The listing builds one solid part. Answer for the finished solid, in the listing's coordinates (mm). A direction names the side the tool comes from. Give positions to 0.01 mm unless a question says otherwise; leave off trailing zeros. Order: outer loops, then holes, each group sorted by start corner. A loop starts at its lowest first (then second) coordinate and runs counter-clockwise, first axis right, second up. Notation, with made-up numbers: (56.25, 1.25) - (91.25, 1.25) arc R21 ccw to (91.25, 22.25) - close; hole circle Ø7 at (52, -4). An arc over 180 degrees is marked (long way). Answer in a Markdown table with one row per item. Add a question column.
```python
from build123d import *

# Parameters (mm, degrees)
AUFSATZ_LINEAR_AUSTRAGEN1_DEPTH = 50
SKIZZE3_R                       = 1.25
SKIZZE3_R_2                     = 1.5
SCHNITT_LINEAR_AUSTRAGEN1_DEPTH = 3
SKIZZE4_W                       = 5
SKIZZE4_H                       = 44
SCHNITT_LINEAR_AUSTRAGEN2_DEPTH = 27
SKIZZE5_R                       = 2.5
SCHNITT_LINEAR_AUSTRAGEN3_DEPTH = 28
SKIZZE6_R                       = 1.25
SCHNITT_LINEAR_AUSTRAGEN4_DEPTH = 3
SKIZZE7_W                       = 5
SKIZZE7_H                       = 15
SCHNITT_LINEAR_AUSTRAGEN5_DEPTH = 3


with BuildPart() as part:
    # Skizze2 → Aufsatz-Linear austragen1 (new body)
    with BuildSketch(Plane.XY):
        Polygon((-4.170146195, 14.050114253), (-21.49065427, -15.949885747), (13.50934573, -15.949885747), (13.50934573, 14.050114253), align=None)
        Polygon((5.50934573, -12.949885747), (-16.294501848, -12.949885747), (-2.438095387, 11.050114253), (5.50934573, 11.050114253), align=None, mode=Mode.SUBTRACT)
    extrude(amount=AUFSATZ_LINEAR_AUSTRAGEN1_DEPTH)

    # Skizze3 → Schnitt-Linear austragen1 (cut)
    with BuildSketch(Plane.XZ.offset(15.949885747)):
        with Locations((11.00934573, 40)):
            Circle(SKIZZE3_R)
        with Locations((11.00934573, 10)):
            Circle(SKIZZE3_R)
        with Locations((1.00934573, 41.25)):
            Circle(SKIZZE3_R_2)
        with Locations((1.00934573, 8.75)):
            Circle(SKIZZE3_R_2)
    extrude(amount=-SCHNITT_LINEAR_AUSTRAGEN1_DEPTH, mode=Mode.SUBTRACT)

    # Skizze4 → Schnitt-Linear austragen2 (cut)
    with BuildSketch(Plane(origin=(0, 14.050114253, 0), x_dir=(1, 0, 0), z_dir=(0, 1, 0))):
        with Locations((11.00934573, -25)):
            Rectangle(SKIZZE4_W, SKIZZE4_H)
    extrude(amount=-SCHNITT_LINEAR_AUSTRAGEN2_DEPTH, mode=Mode.SUBTRACT)

    # Skizze5 → Schnitt-Linear austragen3 (cut)
    with BuildSketch(Plane(origin=(0, 14.050114253, 0), x_dir=(1, 0, 0), z_dir=(0, 1, 0))):
        with Locations((1.00934573, -41.25)):
            Circle(SKIZZE5_R)
        with Locations((1.00934573, -8.75)):
            Circle(SKIZZE5_R)
    extrude(amount=-SCHNITT_LINEAR_AUSTRAGEN3_DEPTH, mode=Mode.SUBTRACT)

    # Skizze6 → Schnitt-Linear austragen4 (cut)
    with BuildSketch(Plane(origin=(-9.21148758, 5.318254834, 0), x_dir=(0, 0, 1), z_dir=(-0.866025404, 0.5, 0))):
        with Locations((35, -1.917317229)):
            Circle(SKIZZE6_R)
        with Locations((15, -1.917317229)):
            Circle(SKIZZE6_R)
    extrude(amount=-SCHNITT_LINEAR_AUSTRAGEN4_DEPTH, mode=Mode.SUBTRACT)

    # Skizze7 → Schnitt-Linear austragen5 (cut)
    with BuildSketch(Plane(origin=(-9.21148758, 5.318254834, 0), x_dir=(0, 0, 1), z_dir=(-0.866025404, 0.5, 0))):
        with Locations((47.5, -7.05833338)):
            Rectangle(SKIZZE7_W, SKIZZE7_H)
        with Locations((2.5, -7.05833338)):
            Rectangle(SKIZZE7_W, SKIZZE7_H)
    extrude(amount=-SCHNITT_LINEAR_AUSTRAGEN5_DEPTH, mode=Mode.SUBTRACT)


solid = part.part
```
(1) Each of these flat-tipped pins is pushed along its axis until it touches: P1, Ø6, axis at x = -12, z = 29, coming from the +Y side; P2, Ø4, axis at y = 8, z = 40, coming from the -X side; P3, Ø2.5, axis at x = 1.5, z = 41.5, coming from the +Y side. Where does it stop, or does it pass through?
(2) Straight lines are drawn through the part: line 1 (Y direction, x = 1, z = 5.5); line 2 (X direction, y = -14, z = 41); line 3 (Z direction, x = 12, y = 9). For each, find the intervals that lie inside material, in ascending order.
(3) Find section A-A, the plane z = 29. Write down the section's boundary in (x, y), plus the area to 3 significant figures.
(4) Find section D-D, the plane x = 0.5. Give the number of separate pieces and of enclosed holes in the cut face, plus the area to 3 significant figures.
(5) Find section B-B, the plane y = -3. Write down the section's boundary in (x, z), plus the area to 3 significant figures.
(6) For faces 4 (the face through (-7.71, 4.96, 2.47)), 5 (the face through (0.47, -13.44, 43.69)), 6 (the face through (-15.21, -8.03, 2.47)), 7 (the face through (-7.71, 4.96, 47.46)), 8 (the face through (-9.463, -1.118, 24.65)), determine the directions among +Z, -Z, +X, -X, +Y, -Y from which every point of the face is accessible in a straight line to the end or side of a thin tool.
(7) Find section C-C, the plane x = 10.5. Write down the section's boundary in (y, z).
(8) The mould has two halves that part along X. Classify faces 1 (the face through (11, 1, 47)), 2 (the face through (13.509, -13.2, 24.9)), 3 (the face through (0.684, -14.964, 7.286)): +X half, -X half, draft (parallel to the pull), parting line (faces both ways), or undercut.
Answer key:
| question | item | result |
|---|---|---|
| 1 | P1 | y = 5.68 |
| 1 | P2 | x = -8.82 |
| 1 | P3 | y = -13.95 |
| 2 | line 1 | -15.95 to -12.95, 11.05 to 14.05 |
| 2 | line 2 | -20.36 to -0.47, 2.49 to 10.26, 11.76 to 13.51 |
| 2 | line 3 | 0 to 3, 47 to 50 |
| 3 | outline | (-21.49, -15.95) - (13.51, -15.95) - (13.51, -12.95) - (8.51, -12.95) - (8.51, 14.05) - (-4.17, 14.05) - close; hole (-16.29, -12.95) - (5.51, -12.95) - (5.51, 11.05) - (-2.44, 11.05) - close |
| 3 | area | 298 mm² |
| 4 | separate pieces | 6 |
| 4 | enclosed holes | 0 |
| 4 | area | 250 mm² |
| 5 | outline | (-14.01, 5) - (-10.55, 5) - (-10.55, 45) - (-14.01, 45) - close; (5.51, 0) - (13.51, 0) - (13.51, 3) - (8.51, 3) - (8.51, 47) - (13.51, 47) - (13.51, 50) - (5.51, 50) - close |
| 5 | area | 319 mm² |
| 6 | face 4 | -Z, -X |
| 6 | face 5 | +Y |
| 6 | face 6 | -Z, +Y |
| 6 | face 7 | +Z, -X |
| 6 | face 8 | +Z, -Z |
| 7 | outline | (-15.95, 0) - (14.05, 0) - (14.05, 3) - (-12.95, 3) - (-12.95, 8.86) - (-15.95, 8.86) - close; (-15.95, 11.14) - (-12.95, 11.14) - (-12.95, 38.86) - (-15.95, 38.86) - close; (-15.95, 41.14) - (-12.95, 41.14) - (-12.95, 47) - (14.05, 47) - (14.05, 50) - (-15.95, 50) - close |
| 8 | face 1 | draft |
| 8 | face 2 | +X half |
| 8 | face 3 | undercut |
